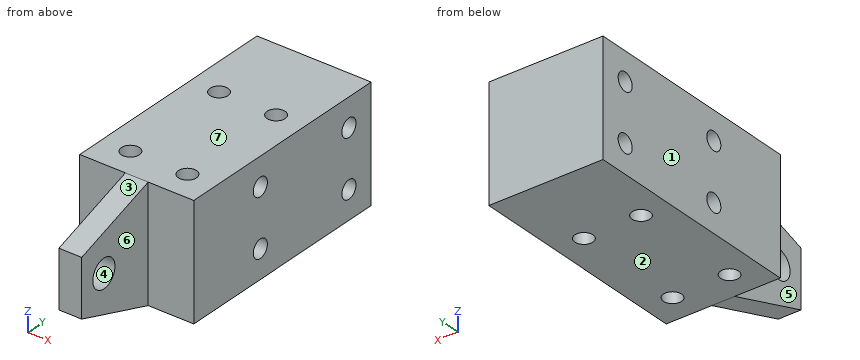
Solid Edge part; units mm, degrees
sketch "Sketch1" plane through (0, 0, 0) normal (0, -1, 0) x (1, 0, 0)
  line L0 (-92.067, 25.1901) -> (-52.067, 25.1901)
  line L1 (-52.067, 25.1901) -> (-52.067, 65.1901)
  line L2 (-52.067, 65.1901) -> (-92.067, 65.1901)
  line L3 (-92.067, 65.1901) -> (-92.067, 25.1901)
  dimension "D1" = 52.067
  dimension "D2" = 52.067
extrude "Protrusion1" add sketch "Sketch1" along normal blind 80
sketch "Sketch2" plane through (-68.067, -75, 45.1901) normal (1, 0, 0) x (0, 1, 0)
  circle A0 centre (-25, 0) radius 5
  line L0 (-5, 20) -> (-35, 10)
  line L1 (-35, 10) -> (-35, -10)
  line L2 (-35, -10) -> (-5, -20)
  line L3 (-5, -20) -> (-5, 20)
  dimension "D1" = 35
  dimension "D2" = 25
extrude "ExtrudedProtrusion_2" add sketch "Sketch2" against normal blind 8
hole "Hole_1" at (-92.067, -50, 55.1901) direction (1, 0, 0) diameter 6.35 end up to next
hole "Hole1" at (-92.067, -10, 35.1901) direction (1, 0, 0) diameter 6.35 end up to next
hole "Hole2" at (-92.067, -50, 35.1901) direction (1, 0, 0) diameter 6.35 end up to next
hole "Hole3" at (-92.067, -10, 55.1901) direction (1, 0, 0) diameter 6.35 end up to next
hole "Hole_5" at (-62.067, -30, 65.1901) direction (0, 0, -1) diameter 6.35 end up to next
hole "Hole4" at (-82.067, -30, 65.1901) direction (0, 0, -1) diameter 6.35 end up to next
hole "Hole5" at (-82.067, -70, 65.1901) direction (0, 0, -1) diameter 6.35 end up to next
hole "Hole6" at (-62.067, -70, 65.1901) direction (0, 0, -1) diameter 6.35 end up to next
properties material "Aluminum, 6061-T6"
Model file for the job. Use its own axes, mm. Face numbers are marked on the shaded views. A direction names the side the tool comes from. Give positions to 0.01 mm unless a question says otherwise; leave off trailing zeros. Write each loop counter-clockwise with the first axis right and the second up, starting at its lowest first coordinate (ties: lowest second). Pieces come first, ordered by that corner, then holes. Notation, with made-up numbers: (38, 55.5) - (80, 55.5) arc R18 cw to (80, 72.5) - close; hole circle Ø11 at (-15, 64.25). An arc over 180 degrees is marked (long way). One line per question, with ' | ' between items. Start each with the question number.
(1) Two-plate mould, pull along Z, no slides. Class the marked faces 1, 2, 3 and 4: +Z half, -Z half, draft (parallel to the pull), parting line (faces both ways), or undercut.
(2) Wall check: line 1 along Y through (x, z) = (-82, 48); line 2 along X through (y, z) = (-70, 44); line 3 along Y through (x, z) = (-83, 53.5). Give the ranges that are in metal, low to high. Write a range as from..to.
(3) 3-axis set-ups, long thin cutter, end or side, ignore diameter. For the marked faces 5, 6 and 7: which of +Z, -Z, +X, -X, +Y, -Y reach the whole face in a straight line?
(4) Slice it at D-D on y = -100. Write the cut outline in (x, z), plus the area to 3 significant figures.
(5) Slice it at B-B on y = -30. Write the cut outline in (x, z).
(6) Slice it at A-A on x = -81. Write the cut outline in (y, z) (3 decimals).
(7) Slice it at C-C on z = 30. Write the cut outline in (x, y) (3 decimals), plus the area to 3 significant figures.
(8) Pin check, flat tips, straight feed: P1, Ø10, axis at x = -82.5, z = 58, coming from the -Y side; P2, Ø9, axis at y = -99.5, z = 42, coming from the +X side. Stop position of each tip, or through.
Results below:
1) face 1: draft | face 2: -Z half | face 3: +Z half | face 4: undercut
2) line 1: -80..-73.17, -66.83..-33.17, -26.83..0 | line 2: -92.07..-85.24, -78.89..-65.24, -58.89..-52.07 | line 3: -80..-73.03, -66.97..-52.69, -47.31..-33.03, -26.97..-12.69, -7.31..0
3) face 5: +Z, -Z, -X, -Y | face 6: +Z, -Z, +X, -Y | face 7: +Z, +X, -X, +Y, -Y
4) outline: (-76.07, 31.86) - (-68.07, 31.86) - (-68.07, 40.19) - (-76.07, 40.19) - close; (-76.07, 50.19) - (-68.07, 50.19) - (-68.07, 58.52) - (-76.07, 58.52) - close | area: 133 mm^2
5) outline: (-92.07, 25.19) - (-85.24, 25.19) - (-85.24, 65.19) - (-92.07, 65.19) - close; (-78.89, 25.19) - (-65.24, 25.19) - (-65.24, 65.19) - (-78.89, 65.19) - close; (-58.89, 25.19) - (-52.07, 25.19) - (-52.07, 65.19) - (-58.89, 65.19) - close
6) outline: (-80, 25.19) - (-72.99, 25.19) - (-72.99, 65.19) - (-80, 65.19) - close; (-67.01, 25.19) - (-32.99, 25.19) - (-32.99, 65.19) - (-67.01, 65.19) - close; (-27.01, 25.19) - (0, 25.19) - (0, 65.19) - (-27.01, 65.19) - close; hole circle Ø6.35 at (-50, 35.19); hole circle Ø6.35 at (-50, 55.19); hole circle Ø6.35 at (-10, 35.19); hole circle Ø6.35 at (-10, 55.19)
7) outline: (-92.067, -80) - (-76.067, -80) - (-76.067, -94.43) - (-68.067, -94.43) - (-68.067, -80) - (-52.067, -80) - (-52.067, 0) - (-92.067, 0) - close; hole circle Ø6.35 at (-82.067, -70); hole circle Ø6.35 at (-82.067, -30); hole circle Ø6.35 at (-62.067, -70); hole circle Ø6.35 at (-62.067, -30) | area: 3,190 mm^2
8) P1: y = -80 | P2: x = -68.07
